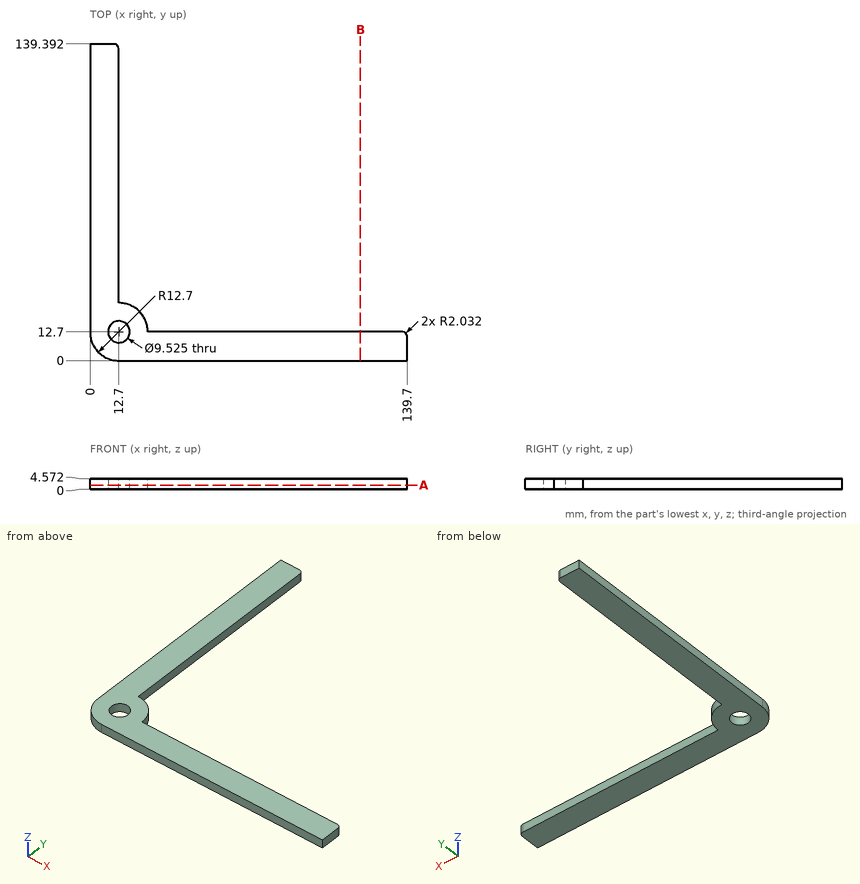
Answer from the drawing. Dimensions are ordinates in mm from the lowest x, y and z of the part. Give positions to 0.01 mm unless a question says otherwise; leave off trailing zeros. Loops run counter-clockwise (first coordinate to the right, second up) from the corner with the lowest first, then second, coordinate; pieces in that order, holes last. Notation, with made-up numbers: (17.5, -9) -> (23.5, -9) arc R13 cw to (23.5, 0) -> close; hole circle Ø1 at (-28, -12). An arc over 180 degrees is marked (long way). Use a Markdown table: item, result.
Q1. Section B-B, the plane x = 119 is taken. Determine the outline of the cut face in (y, z).
Solved:
| item | result |
|---|---|
| outline | (0, 0) -> (12.7, 0) -> (12.7, 4.57) -> (0, 4.57) -> close |
Q2. Section A-A, the plane z = 1.7 is taken. Determine the outline of the cut face in (x, y) (1 decimal).
Solved:
| item | result |
|---|---|
| outline | (0, 12.7) arc R12.7 ccw to (12.7, 0) -> (139.7, 0) -> (139.7, 10.7) arc R2 ccw to (137.7, 12.7) -> (25.4, 12.7) arc R12.7 ccw to (12.7, 25.4) -> (12.7, 137.4) arc R2 ccw to (10.7, 139.4) -> (0, 139.4) -> close; hole circle Ø9.5 at (12.7, 12.7) |
Q3. This flat-tipped pin is pushed along its axis until it touches: pin 1 (4 mm diameter, centred on x = 15, y = 108, fed in from -Z). Where does it stop, or does it pass through?
Solved:
| item | result |
|---|---|
| pin 1 | passes through |
Q4. Find the intervals of material crossed by line 1 along X through (y, z) = (41.5, 3.6); line 2 along X through (y, z) = (19.5, 4.15), in increasing order.
Solved:
| item | result |
|---|---|
| line 1 | x = 0 to 12.7 |
| line 2 | x = 0 to 23.43 |
